Build history of the part. All positions in model axes, mm. Face numbers are marked on the shaded views. A direction names the side the tool comes from. Give positions to 0.01 mm unless a question says otherwise; leave off trailing zeros. Write each loop counter-clockwise with the first axis right and the second up, starting at its lowest first coordinate (ties: lowest second). Pieces come first, ordered by that corner, then holes. Notation, with made-up numbers: (42, -16) -> (89, -16) arc R30 ccw to (89, 19) -> close; hole circle Ø7 at (-30, 40). An arc over 180 degrees is marked (long way). Put each result on its own line as item: value.
from build123d import *

# Parameters (mm, degrees)
SKETCH_1_R            = 57
EXTRUDE_1_DEPTH       = 41
EXTRUDE_START         = -15
EXTRUDE_3_DEPTH       = 15
SKETCH_5_R            = 40
CUT_EXTRUDE_1_DEPTH   = 1
SKETCH_6_R            = 51
SKETCH_7_R            = 45
SKETCH_8_R            = 20
CUT_EXTRUDE_2_DEPTH   = 102.524824572
F_3_0MM_1_D           = 3
F_3_0MM_1_DEPTH       = 7
F_3_0MM_1_CSINK_D     = 11
F_3_0MM_1_CSINK_ANGLE = 90
F_3_0MM_1_TIP         = 0.901290929
FILLET_2_R            = 10
EXTRUDE_START_2       = 62
SKETCH_14_R           = 18
EXTRUDE_4_DEPTH       = 17
SKETCH_15_R           = 11
CUT_EXTRUDE_3_DEPTH   = 1
CUT_EXTRUDE_4_REACH   = 150.883
SKETCH_16_R           = 9
SWEEP_1_PROFILE_R     = 3


with BuildPart() as part:
    # 草图1 → 凸台-拉伸1 (new body)
    with BuildSketch(Plane.XY):
        Circle(SKETCH_1_R)
    extrude(amount=EXTRUDE_1_DEPTH)

    # 草图4 → 凸台-拉伸3 (add)
    with BuildSketch(Plane.XY.offset(41).offset(EXTRUDE_START)):
        with BuildLine():
            Line((19, 62), (19, 60.398675482))
            ThreePointArc((19, 60.398675482), (20.53585261, 55.073432863), (24.671641791, 51.383947798))
            ThreePointArc((24.671641791, 51.383947798), (0, -57), (-24.671641791, 51.383947798))
            ThreePointArc((-24.671641791, 51.383947798), (-20.53585261, 55.073432863), (-19, 60.398675482))
            Line((-19, 60.398675482), (-19, 62))
            ThreePointArc((-19, 62), (0, 81), (19, 62))
        make_face()
    extrude(amount=EXTRUDE_3_DEPTH)

    # 草图5 → 切除-拉伸1 (cut)
    with BuildSketch(Plane.XY.offset(26)):
        with Locations((0, 100)):
            Circle(SKETCH_5_R)
    extrude(amount=CUT_EXTRUDE_1_DEPTH, mode=Mode.SUBTRACT)

    # 草图6 → 切除-放样1 section 0
    with BuildSketch(Plane(origin=(0, 0, 0), x_dir=(-1, 0, 0), z_dir=(0, 0, -1))):
        Circle(SKETCH_6_R)
    # 草图7 → 切除-放样1 section 1
    with BuildSketch(Plane(origin=(0, 0, 22.3), x_dir=(-1, 0, 0), z_dir=(0, 0, -1))):
        Circle(SKETCH_7_R)
    loft(mode=Mode.SUBTRACT)

    # 草图8 → 切除-拉伸2 (cut, through all)
    with BuildSketch(Plane(origin=(0, 0, 22.3), x_dir=(-1, 0, 0), z_dir=(0, 0, -1))):
        Circle(SKETCH_8_R)
    extrude(amount=-CUT_EXTRUDE_2_DEPTH, mode=Mode.SUBTRACT)

    # 草图10 → 切除-旋转1 (revolve, cut)
    with BuildSketch(Plane(origin=(0, 0, 0), x_dir=(0, 0, -1), z_dir=(1, 0, 0)), mode=Mode.PRIVATE) as cut_revolve_1_sk:
        Polygon((-41, 0), (-41, 25.5), (-27, 22), (-27, 0), align=None)
    revolve(cut_revolve_1_sk.sketch.rotate(Axis((0, 0, 0), (0, 0, 1)), 25.647663546), axis=Axis((0, 0, 0), (0, 0, 1)), mode=Mode.SUBTRACT)

    # Ø3.0mm 暗销孔1
    with Locations(Plane.XY.offset(41)):
        with Locations((0, 62)):
            CounterSinkHole(F_3_0MM_1_D / 2, F_3_0MM_1_CSINK_D / 2, depth=F_3_0MM_1_DEPTH, counter_sink_angle=F_3_0MM_1_CSINK_ANGLE)
            with Locations((0, 0, -(F_3_0MM_1_DEPTH + F_3_0MM_1_TIP / 2))):  # 118° drill point
                Cone(0, F_3_0MM_1_D / 2, F_3_0MM_1_TIP, mode=Mode.SUBTRACT)

    # 圆角2
    fillet_2_edges = [part.edges().sort_by_distance(p)[0] for p in [
        (-30.35388293, -48.245640125, 41),
        (20.53585261, 55.073432863, 41),
        (19, 61.199337741, 41),
        (0, 81, 41),
        (-19, 61.199337741, 41),
        (-20.53585261, 55.073432863, 41),
    ]]
    fillet(fillet_2_edges, radius=FILLET_2_R)

    # 草图14 → 凸台-拉伸4 (add)
    with BuildSketch(Plane(origin=(0, 0, 0), x_dir=(0, 0, -1), z_dir=(1, 0, 0)).offset(EXTRUDE_START_2)):
        with Locations((-12, 0)):
            Circle(SKETCH_14_R)
    extrude_4 = extrude(amount=-EXTRUDE_4_DEPTH)

    # 草图15 → 切除-拉伸3 (cut)
    with BuildSketch(Plane(origin=(62, 0, 0), x_dir=(0, 0, -1), z_dir=(1, 0, 0))):
        with Locations((-12, 0)):
            Circle(SKETCH_15_R)
    cut_extrude_3 = extrude(amount=-CUT_EXTRUDE_3_DEPTH, mode=Mode.SUBTRACT)

    # 草图16 → 切除-拉伸4 (cut, up to next)
    with BuildSketch(Plane(origin=(61, 0, 0), x_dir=(0, 0, -1), z_dir=(1, 0, 0)), mode=Mode.PRIVATE) as cut_extrude_4_sk1:
        with Locations((-12, 0)):
            Circle(SKETCH_16_R)
    cut_extrude_4_tool1 = extrude(cut_extrude_4_sk1.sketch, amount=-CUT_EXTRUDE_4_REACH, mode=Mode.PRIVATE) & part.part
    cut_extrude_4 = cut_extrude_4_tool1.solids().sort_by_distance((61, 0, 12))[0]
    add(cut_extrude_4, mode=Mode.SUBTRACT)

    # 镜向2: 凸台-拉伸4, 切除-拉伸3, 切除-拉伸4 across plane
    add(extrude_4.mirror(Plane(origin=(0, 0, 0), x_dir=(0, 0, 1), z_dir=(1, 0, 0))))
    add(cut_extrude_3.mirror(Plane(origin=(0, 0, 0), x_dir=(0, 0, 1), z_dir=(1, 0, 0))), mode=Mode.SUBTRACT)
    add(cut_extrude_4.mirror(Plane(origin=(0, 0, 0), x_dir=(0, 0, 1), z_dir=(1, 0, 0))), mode=Mode.SUBTRACT)

    # 扫描1: sweep along a path in 草图17
    with BuildLine(Plane(origin=(0, 0, 0), x_dir=(0, 0, -1), z_dir=(1, 0, 0))) as sweep_1_path:
        Line((-43.1, -50.6), (-35.054731359, -48.88992536))
    # 扫描1 profile (on start of the path) → 扫描1 (sweep)
    with BuildSketch(Plane(origin=(0, -50.6, 43.1), x_dir=(0, -0.9781476007338048, -0.20791169081776342), z_dir=(0, 0.20791169081776342, -0.9781476007338048))):
        Circle(SWEEP_1_PROFILE_R)
    sweep(path=sweep_1_path.line)


solid = part.part
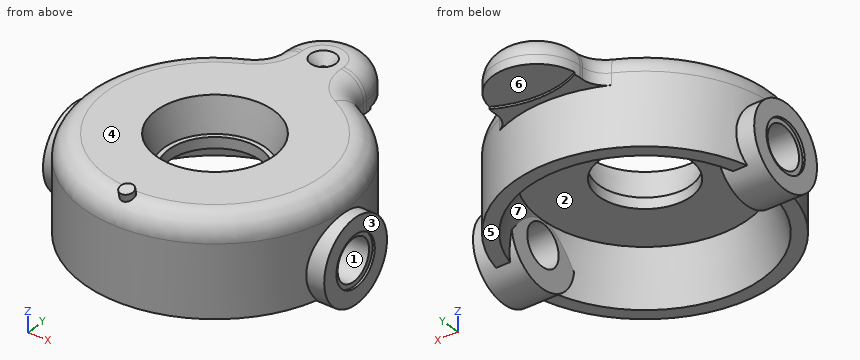
1) Pin check, flat tips, straight feed: pin 1 (0.5 mm diameter, centred on y = 61, z = 27.5, fed in from -X); pin 2 (17.5 mm diameter, centred on y = 0, z = 12, fed in from -X); pin 3 (4 mm diameter, centred on y = 32, z = 29, fed in from -X); pin 4 (1.5 mm diameter, centred on x = 28.5, z = 3, fed in from +Y). Stop position of each tip, or through.
Filled sheet:
pin 1: x = -19
pin 2: through
pin 3: x = -48.47
pin 4: y = 49.79
2) Slice it at A-A (z = 12). Write the cut outline in (x, y), plus the area to 3 significant figures.
Filled sheet:
outline: (-62, -18) -> (-54.08, -18) arc R57 ccw to (54.08, -18) -> (62, -18) -> (62, -11) -> (61, -11) -> (61, -9) -> (45, -9) -> (45, -16.03) arc R47.77 cw to (-45, -16.03) -> (-45, -9) -> (-61, -9) -> (-61, -11) -> (-62, -11) -> close; (-62, 11) -> (-61, 11) -> (-61, 9) -> (-45, 9) -> (-45, 16.03) arc R47.77 cw to (45, 16.03) -> (45, 9) -> (61, 9) -> (61, 11) -> (62, 11) -> (62, 18) -> (54.08, 18) arc R57 ccw to (-54.08, 18) -> (-62, 18) -> close
area: 2,970 mm2
3) Wall check: L1, parallel to X at y = 9, z = 9; L2, parallel to Y at x = -56, z = 12; L3, parallel to X at y = 12.5, z = 2. Give the ranges that are in metal, low to high.
Filled sheet:
L1: -61 to -45, 45 to 61
L2: -18 to -9, 9 to 18
L3: -62 to -45, 45 to 62
4) Tool access for the marked faces 4, 5, 6 and 7: list every direction of +Z, -Z, +X, -X, +Y, -Y with a clear straight run to the whole face (end or side of a thin tool).
Filled sheet:
face 4: +Z, +X, -X, +Y
face 5: -Z, +X, -X, +Y
face 6: -Z, +Y
face 7: -Z
5) Pull direction Z, two halves, no side cores. Call the marked faces 1, 2 and 3: released by +Z, released by -Z, zero draft, split by the parting line, or undercut.
Filled sheet:
face 1: undercut
face 2: released by -Z
face 3: zero draft
